Can you work these out from the model? Positions are in its coordinate system, mm. A direction names the side the tool comes from. Round coordinates to 2 decimals unless told otherwise and drop trailing zeros. Order: outer loops, then holes, each group sorted by start corner. A loop starts at its lowest first (then second) coordinate and runs counter-clockwise, first axis right, second up.
Q1. If we section it at A-A (y = 56.5): Please give me the cut outline in (x, z), plus the area to 3 significant figures.
Q2. If I drill on line 1 (Z direction, x = -34, y = 47); line 2 (X direction, y = 33.5, z = 5.5), over which ranges is the centre line in solid material (lowest first)?
Q3. If we section it at C-C (z = 5.75): Please give me the cut outline in (x, y), plus the area to 3 significant figures.
Q4. For faces 1 (the face through (-51.164, 40, 3)), 2 (the face through (-34, 39, 5)), 3 (the face through (-49, 40, 5)), which set-ups out of +Z, -Z, +X, -X, +Y, -Y let a thin tool reach every point of the face, with its end or its side?
Q5. Will these pins go through, and if not, where does the flat tip stop? P1, Ø8, axis at x = -42, y = 54, coming from the -Z side; P2, Ø4, axis at x = -33.5, y = 33, coming from the +Z side; P3, Ø2.5, axis at y = 46.5, z = 8.5, coming from the -X side; P4, Ø4, axis at y = 44, z = 8, coming from the +X side.
Q6. If we section it at B-B (x = -48): Please give me the cut outline in (y, z).
from build123d import *

# Parameters (mm, degrees)
F0_W     = 10
F0_H     = 50
F1_DEPTH = 10
F2_W     = 50
F2_H     = 5
F3_DEPTH = 5
F4_W     = 50
F4_H     = 5
F5_DEPTH = 5


with BuildPart() as f1:
    # F0 (on Top) → F1 (new body)
    with BuildSketch(Plane.XY):
        with Locations((-41.163797, 39.292196)):
            Rectangle(F0_W, F0_H)
    extrude(amount=F1_DEPTH)

    # F2 (on face) → F3 (join)
    with BuildSketch(Plane.YZ.offset(-36.163797)):
        with Locations((39.292196, 2.5)):
            Rectangle(F2_W, F2_H)
    extrude(amount=F3_DEPTH)

    # F4 (on face) → F5 (join)
    with BuildSketch(Plane(origin=(-46.163797, 0, 0), x_dir=(0, -1, 0), z_dir=(-1, 0, 0))):
        with Locations((-39.292196, 2.5)):
            Rectangle(F4_W, F4_H)
    extrude(amount=F5_DEPTH)


solid = f1.part
Solution:
1. outline: (-51.16, 0) - (-31.16, 0) - (-31.16, 5) - (-36.16, 5) - (-36.16, 10) - (-46.16, 10) - (-46.16, 5) - (-51.16, 5) - close
1. area: 150 mm2
2. line 1: z = 0 to 5
2. line 2: x = -46.16 to -36.16
3. outline: (-46.16, 14.29) - (-36.16, 14.29) - (-36.16, 64.29) - (-46.16, 64.29) - close
3. area: 500 mm2
4. face 1: +Z, -Z, -X, +Y, -Y
4. face 2: +Z, +X, +Y, -Y
4. face 3: +Z, -X, +Y, -Y
5. P1: stops at z = 0
5. P2: stops at z = 5
5. P3: stops at x = -46.16
5. P4: stops at x = -36.16
6. outline: (14.29, 0) - (64.29, 0) - (64.29, 5) - (14.29, 5) - close
